```python
from build123d import *

# Parameters (mm, degrees)
BOSS_EXTRUDE2_DEPTH     = 609.6
CUT_EXTRUDE1_DEPTH      = 1013.46
F_6_32_TAPPED_HOLE1_D   = 2.7051
F_6_32_TAPPED_HOLE2_D   = 2.7051
CUT_EXTRUDE4_DEPTH      = 611.921484317
CUT_EXTRUDE4_DEPTH_BACK = 611.921484317
SKETCH13_W              = 69.85
SKETCH13_H              = 15.24


with BuildPart() as part:
    # Sketch3 → Boss-Extrude2 (new, symmetric)
    with BuildSketch(Plane.XY):
        Polygon((-19.05, 12.7), (-19.05, -12.7), (19.05, -12.7), (19.05, 12.7), (15.875, 12.7), (15.875, -9.525), (-15.875, -9.525), (-15.875, 12.7), align=None)
    extrude(amount=BOSS_EXTRUDE2_DEPTH, both=True)

    # Sketch5 → Cut-Extrude1 (cut)
    with BuildSketch(Plane.XY.offset(609.6)):
        Polygon((-19.05, 12.7), (-15.875, 12.7), (-15.875, -9.525), (15.875, -9.525), (15.875, 12.7), (19.05, 12.7), (19.05, -12.7), (-19.05, -12.7), align=None)
    extrude(amount=-CUT_EXTRUDE1_DEPTH, mode=Mode.SUBTRACT)

    # #6-32 Tapped Hole1 (through all)
    with Locations(Plane.ZY.offset(19.05)):
        with Locations((-601.98, 0)):
            Hole(F_6_32_TAPPED_HOLE1_D / 2)

    # #6-32 Tapped Hole2 (through all)
    with Locations(Plane.ZY.offset(19.05)):
        with Locations((-492.76, 0)):
            Hole(F_6_32_TAPPED_HOLE2_D / 2)

    # Sketch13 → Cut-Extrude4 (cut, two sides: drawn at the far end of the back side and taken through both)
    with BuildSketch(Plane.ZY.offset(19.05).offset(-CUT_EXTRUDE4_DEPTH_BACK)):
        with Locations((-438.785, 5.08)):
            Rectangle(SKETCH13_W, SKETCH13_H)
    extrude(amount=CUT_EXTRUDE4_DEPTH + CUT_EXTRUDE4_DEPTH_BACK, mode=Mode.SUBTRACT)


solid = part.part
```
Work out the finished part from the listing and answer in its coordinate system (mm). A direction names the side the tool comes from. Coordinates: 2 decimals unless noted, no trailing zeros. Order: outer loops, then holes, each group sorted by start corner. A loop starts at its lowest first (then second) coordinate and runs counter-clockwise, first axis right, second up. Notation, with made-up numbers: M 11,-31 L 59,-31 A32 cw 59,5 Z; hole C 59.5,24.25 d6. An arc over 180 degrees is marked long. Use CSV: the item, a comma, the result in double quotes.
1) Consider line 1 (Y direction, x = 18.15, z = -492.76); line 2 (X direction, y = 10.5, z = -594) (3 decimals). Determine where each line is inside the solid, lowest interval first. Write a range as [from, to].
Worked out:
line 1,"y = [-12.7, -1.35], [1.35, 12.7]"
line 2,"x = [-19.05, -15.875], [15.875, 19.05]"
2) Flat-ended cylindrical pins translate along their axes: pin 1 Ø9.5 at (x, z) = (0.5, -545.5) entering from +Y (3 decimals); pin 2 Ø3.5 at (x, y) = (17.5, 3) entering from +Z; pin 3 Ø2 at (y, z) = (0, -601.98) entering from -X; pin 4 Ø1.6 at (x, z) = (17, -437.5) entering from +Y. Find the tip coordinate at first contact, or state that the pin passes through.
Worked out:
pin 1,"stops at y = -9.525"
pin 2,"stops at z = -473.71"
pin 3,"passes through"
pin 4,"stops at y = -2.54"
3) For faces 1 (the face through (0, -9.525, -505)), 2 (the face through (0, -10, -403.86)), 3 (the face through (17, -2.54, -439)), determine the directions among +Z, -Z, +X, -X, +Y, -Y from which every point of the face is accessible in a straight line to the end or side of a thin tool.
Worked out:
face 1,"+Z, -Z, +Y"
face 2,"+Z, +X, -X, +Y, -Y"
face 3,"+Z, +X, -X, +Y"
4) Determine the mould class of faces 4 (the face through (-15.875, 1, -528)), 5 (the face through (15.875, 2, -528)), 6 (the face through (19.05, 0, -528)), 7 (the face through (0, -12.7, -505)) for opening direction X: released by +X, released by -X, zero draft, split by the parting line, or undercut.
Worked out:
face 4,"undercut"
face 5,"undercut"
face 6,"released by +X"
face 7,"zero draft"
5) Section D-D on z = -508 is taken. Write down the section's boundary in (x, y) (3 decimals).
Worked out:
outline,"M -19.05,-12.7 L 19.05,-12.7 L 19.05,12.7 L 15.875,12.7 L 15.875,-9.525 L -15.875,-9.525 L -15.875,12.7 L -19.05,12.7 Z"
6) Section A-A on y = 6 is taken. Write down the section's boundary in (x, z) (3 decimals).
Worked out:
outline,"M -19.05,-609.6 L -15.875,-609.6 L -15.875,-473.71 L -19.05,-473.71 Z; M 15.875,-609.6 L 19.05,-609.6 L 19.05,-473.71 L 15.875,-473.71 Z"
7) Section B-B on z = -452.5 is taken. Write down the section's boundary in (x, y) (3 decimals).
Worked out:
outline,"M -19.05,-12.7 L 19.05,-12.7 L 19.05,-2.54 L 15.875,-2.54 L 15.875,-9.525 L -15.875,-9.525 L -15.875,-2.54 L -19.05,-2.54 Z"
8) Section C-C on x = -13.5 is taken. Write down the section's boundary in (y, z) (3 decimals).
Worked out:
outline,"M -12.7,-609.6 L -9.525,-609.6 L -9.525,-403.86 L -12.7,-403.86 Z"
